Geometry check sheet. Reference: the model listing, model coordinates, mm. Coordinates: 2 decimals unless noted, no trailing zeros. Write each loop counter-clockwise with the first axis right and the second up, starting at its lowest first coordinate (ties: lowest second). Pieces come first, ordered by that corner, then holes. Notation, with made-up numbers: (-4.5, 0.5) -> (50.5, 0.5) arc R18 cw to (50.5, 21.5) -> close; hole circle Ø7 at (58.5, 69). An arc over 180 degrees is marked (long way). Use a Markdown table: item, result.
```python
from build123d import *

# Parameters (mm, degrees)
F0_W     = 19.05
F0_H     = 76.2
F0_W_2   = 63.5
F1_DEPTH = 12.7


with BuildPart() as f1:
    # F0 (on Top) → F1 (new body)
    with BuildSketch(Plane.XY):
        with Locations((-31.324641, 8.143183)):
            Rectangle(F0_W, F0_H)
        Polygon((-31.324641, -4.556817), (-24.974641, -4.556817), (-24.974641, -7.731817), (-24.974641, -10.906817), (-31.324641, -10.906817), (-31.324641, -7.731817), align=None, mode=Mode.SUBTRACT)
        Polygon((-31.324641, 11.318183), (-24.974641, 11.318183), (-24.974641, 8.143183), (-24.974641, 4.968183), (-31.324641, 4.968183), (-31.324641, 8.143183), align=None, mode=Mode.SUBTRACT)
        Polygon((-31.324641, 27.193183), (-24.974641, 27.193183), (-24.974641, 24.018183), (-24.974641, 20.843183), (-31.324641, 20.843183), (-31.324641, 24.018183), align=None, mode=Mode.SUBTRACT)
        with Locations((9.950359, 8.143183)):
            Rectangle(F0_W_2, F0_H)
        Polygon((48.050359, 46.243183), (41.700359, 46.243183), (41.700359, -29.956817), (48.050359, -29.956817), (48.050359, -10.906817), (44.875359, -10.906817), (44.875359, -7.731817), (44.875359, -4.556817), (48.050359, -4.556817), (48.050359, 4.968183), (44.875359, 4.968183), (44.875359, 8.143183), (44.875359, 11.318183), (48.050359, 11.318183), (48.050359, 20.843183), (44.875359, 20.843183), (44.875359, 24.018183), (44.875359, 27.193183), (48.050359, 27.193183), align=None)
        Polygon((60.750359, 46.243183), (48.050359, 46.243183), (48.050359, 27.193183), (51.225359, 27.193183), (51.225359, 24.018183), (51.225359, 20.843183), (48.050359, 20.843183), (48.050359, 11.318183), (51.225359, 11.318183), (51.225359, 8.143183), (51.225359, 4.968183), (48.050359, 4.968183), (48.050359, -4.556817), (51.225359, -4.556817), (51.225359, -7.731817), (51.225359, -10.906817), (48.050359, -10.906817), (48.050359, -29.956817), (60.750359, -29.956817), align=None)
    extrude(amount=F1_DEPTH)


solid = f1.part
```
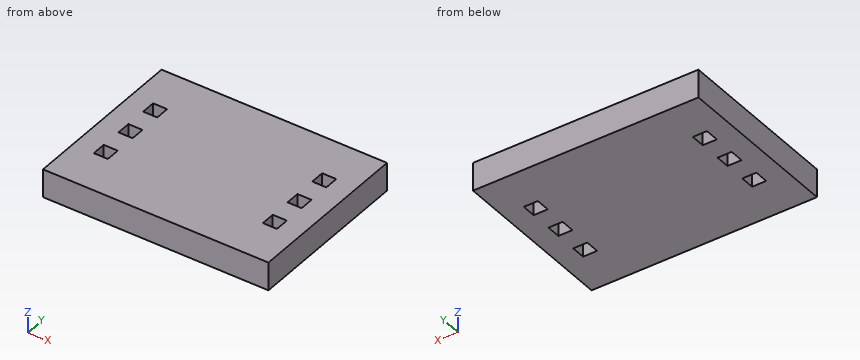
Item 1: Section check B-B on y = 22.5. Record the boundary of the cut face in (x, z), then the cut area to 3 significant figures.
Answer block:
| item | result |
|---|---|
| outline | (-40.85, 0) -> (-31.32, 0) -> (-31.32, 12.7) -> (-40.85, 12.7) -> close; (-24.97, 0) -> (44.88, 0) -> (44.88, 12.7) -> (-24.97, 12.7) -> close; (51.23, 0) -> (60.75, 0) -> (60.75, 12.7) -> (51.23, 12.7) -> close |
| area | 1,130 mm^2 |
Item 2: Section check A-A on x = -29. Record the boundary of the cut face in (y, z), then the cut area to 3 significant figures.
Answer block:
| item | result |
|---|---|
| outline | (-29.96, 0) -> (-10.91, 0) -> (-10.91, 12.7) -> (-29.96, 12.7) -> close; (-4.56, 0) -> (4.97, 0) -> (4.97, 12.7) -> (-4.56, 12.7) -> close; (11.32, 0) -> (20.84, 0) -> (20.84, 12.7) -> (11.32, 12.7) -> close; (27.19, 0) -> (46.24, 0) -> (46.24, 12.7) -> (27.19, 12.7) -> close |
| area | 726 mm^2 |
Item 3: Thickness scan on L1, parallel to Y at x = 45.5, z = 6; L2, parallel to X at y = 11, z = 1.75. Record the ranges inside material, lowest first. Write a range as [from, to].
Answer block:
| item | result |
|---|---|
| L1 | y = [-29.96, -10.91], [-4.56, 4.97], [11.32, 20.84], [27.19, 46.24] |
| L2 | x = [-40.85, -31.32], [-24.97, 44.88], [51.23, 60.75] |
Item 4: Section check C-C on z = 11. Record the boundary of the cut face in (x, y).
Answer block:
| item | result |
|---|---|
| outline | (-40.85, -29.96) -> (60.75, -29.96) -> (60.75, 46.24) -> (-40.85, 46.24) -> close; hole (-31.32, -10.91) -> (-24.97, -10.91) -> (-24.97, -4.56) -> (-31.32, -4.56) -> close; hole (-31.32, 4.97) -> (-24.97, 4.97) -> (-24.97, 11.32) -> (-31.32, 11.32) -> close; hole (-31.32, 20.84) -> (-24.97, 20.84) -> (-24.97, 27.19) -> (-31.32, 27.19) -> close; hole (44.88, -10.91) -> (51.23, -10.91) -> (51.23, -4.56) -> (44.88, -4.56) -> close; hole (44.88, 4.97) -> (51.23, 4.97) -> (51.23, 11.32) -> (44.88, 11.32) -> close; hole (44.88, 20.84) -> (51.23, 20.84) -> (51.23, 27.19) -> (44.88, 27.19) -> close |
